Verification items for the finished model (mm, model axes). A direction names the side the tool comes from. Coordinates: 2 decimals unless noted, no trailing zeros. Write each loop counter-clockwise with the first axis right and the second up, starting at its lowest first coordinate (ties: lowest second). Pieces come first, ordered by that corner, then holes. Notation, with made-up numbers: (37.25, 72.25) -> (83.25, 72.25) arc R26 ccw to (83.25, 103.25) -> close; hole circle Ø7 at (38.5, 87.5). An arc over 180 degrees is marked (long way). Write each question's results on one line, items separated by ' | '. Start each with the question number.
from build123d import *

# Parameters (mm, degrees)
SKETCH1_R           = 22
BOSS_EXTRUDE1_DEPTH = 10
SKETCH2_R           = 28.75
BOSS_EXTRUDE2_DEPTH = 1
SKETCH3_R           = 1.5
CUT_EXTRUDE1_DEPTH  = 1
CUT_EXTRUDE2_DEPTH  = 1
FILLET1_R           = 20
SKETCH5_R           = 4
BOSS_EXTRUDE3_DEPTH = 1
SKETCH6_R           = 1
BOSS_EXTRUDE4_DEPTH = 0.5
SKETCH7_R           = 3
BOSS_EXTRUDE5_DEPTH = 6


with BuildPart() as part:
    # Sketch1 → Boss-Extrude1 (new body)
    with BuildSketch(Plane(origin=(0, 0, 0), x_dir=(1, 0, 0), z_dir=(0, 1, 0))):
        with Locations(Location((0, 0, 0), (0, 0, 270))):
            Circle(SKETCH1_R)
    extrude(amount=BOSS_EXTRUDE1_DEPTH)

    # Sketch2 → Boss-Extrude2 (add)
    with BuildSketch(Plane(origin=(0, 10, 0), x_dir=(1, 0, 0), z_dir=(0, 1, 0))):
        with Locations(Location((0, 0, 0), (0, 0, 270))):
            Circle(SKETCH2_R)
    extrude(amount=BOSS_EXTRUDE2_DEPTH)

    # Sketch3 → Cut-Extrude1 (cut)
    with BuildSketch(Plane(origin=(0, 11, 0), x_dir=(1, 0, 0), z_dir=(0, 1, 0))):
        with Locations(Location((0, -24.75, 0), (0, 0, 270))):
            Circle(SKETCH3_R)
        with Locations(Location((0, 24.75, 0), (0, 0, 270))):
            Circle(SKETCH3_R)
    extrude(amount=-CUT_EXTRUDE1_DEPTH, mode=Mode.SUBTRACT)

    # Sketch4 → Cut-Extrude2 (cut)
    with BuildSketch(Plane.XZ.offset(-10)):
        with BuildLine():
            ThreePointArc((-16.042391304, -23.858000361), (-22, 0), (-16.042391304, 23.858000361))
            ThreePointArc((-16.042391304, 23.858000361), (-28.75, 0), (-16.042391304, -23.858000361))
        make_face()
        with BuildLine():
            ThreePointArc((16.042391304, -23.858000361), (28.75, 0), (16.042391304, 23.858000361))
            ThreePointArc((16.042391304, 23.858000361), (22, 0), (16.042391304, -23.858000361))
        make_face()
    extrude(amount=-CUT_EXTRUDE2_DEPTH, mode=Mode.SUBTRACT)

    # Fillet1
    fillet1_edges = [part.edges().sort_by_distance(p)[0] for p in [
        (-16.042391304, 10.5, 23.858000361),
        (-16.042391304, 10.5, -23.858000361),
        (16.042391304, 10.5, -23.858000361),
        (16.042391304, 10.5, 23.858000361),
    ]]
    fillet(fillet1_edges, radius=FILLET1_R)

    # Sketch5 → Boss-Extrude3 (add)
    with BuildSketch(Plane(origin=(0, 11, 0), x_dir=(1, 0, 0), z_dir=(0, 1, 0))):
        with Locations(Location((0, 0, 0), (0, 0, 270))):
            Circle(SKETCH5_R)
    extrude(amount=BOSS_EXTRUDE3_DEPTH)

    # Sketch6 → Boss-Extrude4 (add)
    with BuildSketch(Plane(origin=(0, 12, 0), x_dir=(1, 0, 0), z_dir=(0, 1, 0))):
        with Locations(Location((0, 0, 0), (0, 0, 270))):
            Circle(SKETCH6_R)
    extrude(amount=BOSS_EXTRUDE4_DEPTH)

    # Sketch7 → Boss-Extrude5 (add)
    with BuildSketch(Plane(origin=(0, 12.5, 0), x_dir=(1, 0, 0), z_dir=(0, 1, 0))):
        with Locations(Location((0, 0, 0), (0, 0, 270))):
            Circle(SKETCH7_R)
    extrude(amount=BOSS_EXTRUDE5_DEPTH)


solid = part.part
1. Depth check by flat-ended pin: pin 1 Ø10 at (x, y) = (-9, 4.5) entering from +Z; pin 2 Ø8 at (y, z) = (11, 17) entering from -X; pin 3 Ø8 at (x, z) = (-8, 9) entering from +Y. Enter the tip coordinate at first touch or a pass-through.
2. Sectioned sample at B-B on y = 1.75. Record the cut outline in (x, z), plus the area to 3 significant figures.
3. Sectioned sample at C-C on y = 17.25. Record the cut outline in (x, z), plus the area to 3 significant figures.
4. Material ranges on probe 1 along Y at (x, z) = (7, 12); probe 2 along X at (y, z) = (2, 0.5); probe 3 along X at (y, z) = (10.75, -24.75), recorded low to high. Write a range as from..to.
5. Mould release check, pull along Y, two halves, no side actions. Record for faces 6 (the cylindrical face through (0.9, 15.46, 2.86)), 7 (the flat face through (1, 12.5, -1)), 8 (the flat face through (0, 18.5, 0)): +Y half, -Y half, draft (parallel to the pull), parting line (faces both ways), or undercut.
6. Tool access check on faces 1 (the cylindrical face through (-0.976, 12.246, -0.217)), 2 (the cylindrical face through (-21.477, 4.93, -4.769)), 3 (the flat face through (0, 10, 23)), 4 (the cylindrical face through (-3.905, 11.493, -0.867)), 5 (the cylindrical face through (0.07, 10.51, 23.25)). Record the directions out of +Z, -Z, +X, -X, +Y, -Y that give a thin tool (end or side, any length) a straight path to the whole face; none if there is none.
7. Sectioned sample at A-A on x = 0. Record the cut outline in (y, z), plus the area to 4 significant figures.
Computed values:
1) pin 1: stops at z = 21.63 | pin 2: stops at x = -20.31 | pin 3: stops at y = 11
2) outline: circle Ø44 at (0, 0) | area: 1,520 mm^2
3) outline: circle Ø6 at (0, 0) | area: 28.3 mm^2
4) probe 1: y = 0..11 | probe 2: x = -21.99..21.99 | probe 3: x = -12.7..-1.5, 1.5..12.7
5) face 6: draft | face 7: undercut | face 8: +Y half
6) face 1: none | face 2: -Y | face 3: +Z, -Y | face 4: +Y | face 5: +Y, -Y
7) outline: (0, -22) -> (10, -22) -> (10, -23.25) -> (11, -23.25) -> (11, -4) -> (12, -4) -> (12, -1) -> (12.5, -1) -> (12.5, -3) -> (18.5, -3) -> (18.5, 3) -> (12.5, 3) -> (12.5, 1) -> (12, 1) -> (12, 4) -> (11, 4) -> (11, 23.25) -> (10, 23.25) -> (10, 22) -> (0, 22) -> close; (10, -28.75) -> (11, -28.75) -> (11, -26.25) -> (10, -26.25) -> close; (10, 26.25) -> (11, 26.25) -> (11, 28.75) -> (10, 28.75) -> close | area: 536.5 mm^2
